Part model, mm, in its own coordinate system. A direction names the side the tool comes from. Coordinates: 2 decimals unless noted, no trailing zeros. Loops run counter-clockwise (first coordinate to the right, second up) from the corner with the lowest first, then second, coordinate; pieces in that order, holes last. Notation, with made-up numbers: (-38, -7.75) -> (19, -7.75) arc R25 ccw to (19, 20.25) -> close; hole circle Ø8 at (-4, -12). An arc over 180 degrees is marked (long way). Use one line per item in the form item = value. Start each with the question number.
(1) Drill centre lines: L1, parallel to X at y = 14, z = -25.25; L2, parallel to X at y = 12, z = -27.5; L3, parallel to Y at x = -68.5, z = -21.5. Where is each one in solid material? Low to high. Write a range as [from, to].
(2) 3-axis set-ups, long thin cutter, end or side, ignore diameter. For faces 1 (the flat face through (-74, 16, -31.991)), 2 (the flat face through (-67, 32, -27)), 3 (the flat face through (-94.449, 15.9, -34.3)), 4 (the cylindrical face through (-37.999, 26.573, -33.324)), 5 (the cylindrical face through (-93.414, 14.509, -29.235)): which of +Z, -Z, +X, -X, +Y, -Y reach the whole face in a straight line?
(3) Mould opens along X. For faces 6 (the flat face through (-37.086, 28, -31)), 7 (the cylindrical face through (-78.405, 16.553, -32.617)), 8 (the flat face through (-93, 8, -33.966)), 9 (the flat face through (-92.349, 16, -27)) say: +X half, -X half, draft (parallel to the pull), parting line (faces both ways), or undercut.
(4) Band-saw the part on A-A on x = -71. Give the cut face in (y, z).
(5) Pin check, flat tip, straight feed: P1, Ø9, axis at x = -54.76, y = 16, coming from the +Z side. Stop position of the tip, or through.
(6) Band-saw the part on D-D on y = 23. Give the cut face in (x, z).
(7) Band-saw the part on C-C on y = 2.5. Give the cut face in (x, z).
(8) Band-saw the part on B-B on y = 16. Count the separate pieces of the cut face and the enclosed holes in it, then the cut area to 3 significant figures.
```python
from build123d import *

# Parameters (mm, degrees)
SKETCH1_W               = 55.5625
SKETCH1_H               = 31.75
BOSS_EXTRUDE1_DEPTH     = 28.575
SKETCH2_R               = 7.62
CUT_EXTRUDE1_DEPTH      = 13.335
CUT_EXTRUDE2_DEPTH      = 12.7
SKETCH4_R               = 1.8415
CUT_EXTRUDE3_DEPTH      = 25.4
CUT_EXTRUDE4_DEPTH      = 17.78
SKETCH6_W               = 55.5625
SKETCH6_H               = 28.575
CUT_EXTRUDE5_DEPTH      = 15.875
SKETCH7_R               = 2.778125
CUT_EXTRUDE7_DEPTH      = 7.9375
SKETCH8_R               = 2.4
BOSS_EXTRUDE2_DEPTH     = 1.8
BOSS_EXTRUDE3_DEPTH     = 4
SKETCH11_W              = 55.5625
SKETCH11_H              = 0.575
CUT_EXTRUDE8_DEPTH      = 102.162047202
CUT_EXTRUDE8_DEPTH_BACK = 102.162047202
SKETCH12_R              = 3.255
SKETCH12_R_2            = 2.45
CUT_EXTRUDE10_DEPTH     = 2.1


with BuildPart() as part:
    # Sketch1 → Boss-Extrude1 (new body)
    with BuildSketch(Plane(origin=(0, 0, 0), x_dir=(1, 0, 0), z_dir=(0, 1, 0))):
        with Locations((-66.667749699, 35.16562105)):
            Rectangle(SKETCH1_W, SKETCH1_H)
    extrude(amount=BOSS_EXTRUDE1_DEPTH)

    # Sketch2 → Cut-Extrude1 (cut)
    with BuildSketch(Plane.XY.offset(-19.29062105)):
        with Locations((-54.761499699, 16)):
            Circle(SKETCH2_R)
    extrude(amount=-CUT_EXTRUDE1_DEPTH, mode=Mode.SUBTRACT)

    # Sketch3 → Cut-Extrude2 (cut)
    with BuildSketch(Plane.XY.offset(-19.29062105)):
        with BuildLine():
            Line((-80.161499699, 20.7625), (-67.461499699, 20.7625))
            ThreePointArc((-67.461499699, 20.7625), (-62.698999699, 16), (-67.461499699, 11.2375))
            Line((-67.461499699, 11.2375), (-80.161499699, 11.2375))
            ThreePointArc((-80.161499699, 11.2375), (-84.923999699, 16), (-80.161499699, 20.7625))
        make_face()
    extrude(amount=-CUT_EXTRUDE2_DEPTH, mode=Mode.SUBTRACT)

    # Sketch4 → Cut-Extrude3 (cut)
    with BuildSketch(Plane.XY.offset(-31.99062105)):
        with Locations((-80.161499699, 16)):
            Circle(SKETCH4_R)
        with Locations((-67.461499699, 16)):
            Circle(SKETCH4_R)
    extrude(amount=-CUT_EXTRUDE3_DEPTH, mode=Mode.SUBTRACT)

    # Sketch5 → Cut-Extrude4 (cut)
    with BuildSketch(Plane(origin=(0, 0, -51.04062105), x_dir=(-1, 0, 0), z_dir=(0, 0, -1))):
        with BuildLine():
            Line((67.461499699, 11.2375), (80.161499699, 11.2375))
            ThreePointArc((80.161499699, 11.2375), (84.923999699, 16), (80.161499699, 20.7625))
            Line((80.161499699, 20.7625), (67.461499699, 20.7625))
            ThreePointArc((67.461499699, 20.7625), (62.698999699, 16), (67.461499699, 11.2375))
        make_face()
    extrude(amount=-CUT_EXTRUDE4_DEPTH, mode=Mode.SUBTRACT)

    # Sketch6 → Cut-Extrude5 (cut)
    with BuildSketch(Plane(origin=(0, 0, -51.04062105), x_dir=(-1, 0, 0), z_dir=(0, 0, -1))):
        with Locations((66.667749699, 14.2875)):
            Rectangle(SKETCH6_W, SKETCH6_H)
    extrude(amount=-CUT_EXTRUDE5_DEPTH, mode=Mode.SUBTRACT)

    # Sketch7 → Cut-Extrude7 (cut)
    with BuildSketch(Plane.XY.offset(-32.62562105)):
        with Locations((-54.761499699, 16)):
            Circle(SKETCH7_R)
    extrude(amount=-CUT_EXTRUDE7_DEPTH, mode=Mode.SUBTRACT)

    # Sketch8 → Boss-Extrude2 (add)
    with BuildSketch(Plane(origin=(-38.886499699, 0, 0), x_dir=(0, 0, -1), z_dir=(1, 0, 0))):
        with Locations(Location((31.16562105, 4, 0), (0, 0, 180))):
            Circle(SKETCH8_R)
        with Locations(Location((23.16562105, 4, 0), (0, 0, 180))):
            Circle(SKETCH8_R)
        with Locations(Location((23.16562105, 11.874, 0), (0, 0, 180))):
            Circle(SKETCH8_R)
        with Locations(Location((31.16562105, 11.874, 0), (0, 0, 180))):
            Circle(SKETCH8_R)
        with Locations(Location((23.16562105, 19.748, 0), (0, 0, 180))):
            Circle(SKETCH8_R)
        with Locations(Location((31.16562105, 19.748, 0), (0, 0, 180))):
            Circle(SKETCH8_R)
        with Locations(Location((23.16562105, 27.622, 0), (0, 0, 156.604030276))):
            Circle(SKETCH8_R)
        with Locations(Location((31.16562105, 27.622, 0), (0, 0, 156.604030276))):
            Circle(SKETCH8_R)
    extrude(amount=BOSS_EXTRUDE2_DEPTH)

    # Sketch10 → Boss-Extrude3 (add)
    with BuildSketch(Plane(origin=(0, 28.575, 0), x_dir=(1, 0, 0), z_dir=(0, 1, 0))):
        Polygon((-38.886499699, 19.29062105), (-38.886499699, 20.962942907), (-38.886499699, 25.368299192), (-38.886499699, 28.962942907), (-38.886499699, 33.368299192), (-38.886499699, 35.16562105), (-94.448999699, 35.16562105), (-94.448999699, 19.29062105), align=None)
    extrude(amount=BOSS_EXTRUDE3_DEPTH)

    # Sketch11 → Cut-Extrude8 (cut, two sides)
    with BuildSketch(Plane.XY.offset(-19.29062105)) as cut_extrude8_sk:
        with Locations((-66.667749699, 32.2875)):
            Rectangle(SKETCH11_W, SKETCH11_H)
    extrude(amount=CUT_EXTRUDE8_DEPTH, mode=Mode.SUBTRACT)
    extrude(cut_extrude8_sk.sketch, amount=-CUT_EXTRUDE8_DEPTH_BACK, mode=Mode.SUBTRACT)

    # Sketch12 → Cut-Extrude10 (cut)
    with BuildSketch(Plane.ZY.offset(94.448999699)):
        Polygon((-33.96562105, 30.8), (-31.46562105, 30.8), (-31.46562105, 30.5), (-30.86562105, 30.5), (-30.86562105, 30.8), (-23.59062105, 30.8), (-23.59062105, 30.5), (-22.99062105, 30.5), (-22.99062105, 30.8), (-20.49062105, 30.8), (-20.49062105, 28.3), (-20.79062105, 28.3), (-20.79062105, 27.7), (-20.49062105, 27.7), (-20.49062105, 20.426), (-20.79062105, 20.426), (-20.79062105, 19.826), (-20.49062105, 19.826), (-20.49062105, 12.552), (-20.79062105, 12.552), (-20.79062105, 11.952), (-20.49062105, 11.952), (-20.49062105, 4.678), (-20.79062105, 4.678), (-20.79062105, 4.078), (-20.49062105, 4.078), (-20.49062105, 1.2), (-22.99062105, 1.2), (-22.99062105, 1.5), (-23.59062105, 1.5), (-23.59062105, 1.2), (-30.86562105, 1.2), (-30.86562105, 1.5), (-31.46562105, 1.5), (-31.46562105, 1.2), (-33.96562105, 1.2), (-33.96562105, 4.078), (-33.66562105, 4.078), (-33.66562105, 4.678), (-33.96562105, 4.678), (-33.96562105, 11.952), (-33.66562105, 11.952), (-33.66562105, 12.552), (-33.96562105, 12.552), (-33.96562105, 19.826), (-33.66562105, 19.826), (-33.66562105, 20.426), (-33.96562105, 20.426), (-33.96562105, 27.7), (-33.66562105, 27.7), (-33.66562105, 28.3), (-33.96562105, 28.3), align=None)
        with Locations((-27.29062105, 24)):
            Circle(SKETCH12_R, mode=Mode.SUBTRACT)
        with Locations((-27.29062105, 16)):
            Circle(SKETCH12_R, mode=Mode.SUBTRACT)
        with Locations((-27.29062105, 8)):
            Circle(SKETCH12_R, mode=Mode.SUBTRACT)
        with Locations((-27.29062105, 8)):
            Circle(SKETCH12_R_2)
        with Locations((-27.29062105, 16)):
            Circle(SKETCH12_R_2)
        with Locations((-27.29062105, 24)):
            Circle(SKETCH12_R_2)
    extrude(amount=-CUT_EXTRUDE10_DEPTH, mode=Mode.SUBTRACT)


solid = part.part
```
A:
q1.L1 = [-94.45, -84.48], [-63.14, -62.11], [-47.41, -38.89]
q1.L2 = [-92.35, -82.75], [-64.88, -61.25], [-48.28, -38.89]
q1.L3 = [0, 11.24], [20.76, 32]
q2.face_1 = +Z
q2.face_2 = +Z, -Z, +X, -X, +Y
q2.face_3 = +Z, -Z, -X, +Y, -Y
q2.face_4 = +X
q2.face_5 = -X
q3.face_6 = +X half
q3.face_7 = undercut
q3.face_8 = draft
q3.face_9 = -X half
q4.outline = (0, -35.17) -> (11.24, -35.17) -> (11.24, -33.26) -> (20.76, -33.26) -> (20.76, -35.17) -> (32, -35.17) -> (32, -19.29) -> (20.76, -19.29) -> (20.76, -31.99) -> (11.24, -31.99) -> (11.24, -19.29) -> (0, -19.29) -> close
q5.P1 = -32.63
q6.outline = (-94.45, -35.17) -> (-38.89, -35.17) -> (-38.89, -19.29) -> (-51.75, -19.29) -> (-51.75, -32.63) -> (-57.77, -32.63) -> (-57.77, -19.29) -> (-94.45, -19.29) -> (-94.45, -20.49) -> (-92.35, -20.49) -> (-92.35, -24.19) -> (-94.45, -24.19) -> (-94.45, -25.05) -> (-92.35, -25.05) -> (-92.35, -29.53) -> (-94.45, -29.53) -> (-94.45, -30.39) -> (-92.35, -30.39) -> (-92.35, -33.97) -> (-94.45, -33.97) -> close
q7.outline = (-94.45, -35.17) -> (-38.89, -35.17) -> (-38.89, -33.04) -> (-37.09, -33.04) -> (-37.09, -29.29) -> (-38.89, -29.29) -> (-38.89, -25.04) -> (-37.09, -25.04) -> (-37.09, -21.29) -> (-38.89, -21.29) -> (-38.89, -19.29) -> (-94.45, -19.29) -> (-94.45, -20.49) -> (-92.35, -20.49) -> (-92.35, -33.97) -> (-94.45, -33.97) -> close
q8.separate_pieces = 4
q8.enclosed_holes = 0
q8.area = 306 mm²
